```python
from build123d import *

# Parameters (mm, degrees)
SKETCH1_R           = 2.5
BOSS_EXTRUDE1_DEPTH = 16
SKETCH2_R           = 1.25
BOSS_EXTRUDE2_DEPTH = 4.5
BOSS_EXTRUDE3_START = 3.5
SKETCH3_R           = 1.25
BOSS_EXTRUDE3_DEPTH = 3.5


with BuildPart() as part:
    # Sketch1 → Boss-Extrude1 (new body)
    with BuildSketch(Plane(origin=(0, 0, 0), x_dir=(1, 0, 0), z_dir=(0, 1, 0))):
        with Locations(Location((0, 0, 0), (0, 0, 270))):
            Circle(SKETCH1_R)
    extrude(amount=BOSS_EXTRUDE1_DEPTH)

    # Sketch2 → Boss-Extrude2 (add)
    with BuildSketch(Plane(origin=(0, 16, 0), x_dir=(1, 0, 0), z_dir=(0, 1, 0))):
        with Locations(Location((0, 0, 0), (0, 0, 270))):
            Circle(SKETCH2_R)
    extrude(amount=BOSS_EXTRUDE2_DEPTH)

    # Sketch3 → Boss-Extrude3 (add)
    with BuildSketch(Plane(origin=(0, 0, 0), x_dir=(-1, 0, 0), z_dir=(0, -1, 0)).offset(BOSS_EXTRUDE3_START)):
        with Locations(Location((0, 0, 0), (0, 0, 270))):
            Circle(SKETCH3_R)
    extrude(amount=-BOSS_EXTRUDE3_DEPTH)


solid = part.part
```
Model file for the job. Use its own axes, mm. A direction names the side the tool comes from. Round coordinates to 2 decimals unless told otherwise and drop trailing zeros. Write each loop counter-clockwise with the first axis right and the second up, starting at its lowest first coordinate (ties: lowest second). Pieces come first, ordered by that corner, then holes. Notation, with made-up numbers: (16.5, 4) -> (24.5, 4) arc R23 ccw to (24.5, 33) -> close; hole circle Ø11 at (19, -3). An arc over 180 degrees is marked (long way). Answer as CSV lines item,"result".
1. Tool access for faces 1 (the face through (1.22, -1.77, -0.27)), 2 (the face through (-2.44, 7.89, -0.54)), 3 (the face through (-1.22, 18.22, -0.27)): list every direction of +Z, -Z, +X, -X, +Y, -Y with a clear straight run to the whole face (end or side of a thin tool).
Resolved:
face 1,"-Y"
face 2,"+Y, -Y"
face 3,"+Y"
2. Slice it at A-A, the plane z = 0. List the corners of the cut face in (x, y), plus the area to 3 significant figures.
Resolved:
outline,"(-2.5, 0) -> (-1.25, 0) -> (-1.25, -3.5) -> (1.25, -3.5) -> (1.25, 0) -> (2.5, 0) -> (2.5, 16) -> (1.25, 16) -> (1.25, 20.5) -> (-1.25, 20.5) -> (-1.25, 16) -> (-2.5, 16) -> close"
area,"100 mm²"
3. Slice it at D-D, the plane y = 19. List the corners of the cut face in (x, z), plus the area to 3 significant figures.
Resolved:
outline,"circle Ø2.5 at (0, 0)"
area,"4.91 mm²"
4. Slice it at C-C, the plane y = 14.5. List the corners of the cut face in (x, z).
Resolved:
outline,"circle Ø5 at (0, 0)"
5. Slice it at B-B, the plane x = 0. List the corners of the cut face in (y, z).
Resolved:
outline,"(-3.5, -1.25) -> (0, -1.25) -> (0, -2.5) -> (16, -2.5) -> (16, -1.25) -> (20.5, -1.25) -> (20.5, 1.25) -> (16, 1.25) -> (16, 2.5) -> (0, 2.5) -> (0, 1.25) -> (-3.5, 1.25) -> close"
6. Drill centre lines: line 1 (Y direction, x = -1.05, z = 1.55); line 2 (Z direction, x = 0.15, y = 9.75); line 3 (X direction, y = 14.75, z = -1.7). Where is each one in solid material? Low to high.
Resolved:
line 1,"0 to 16"
line 2,"-2.5 to 2.5"
line 3,"-1.83 to 1.83"
